Autodesk Fusion 360 part; units mm, degrees
sketch "Sketch3" plane through (0, 0, 0) normal (1, 0, 0) x (0, 1, 0)
  line L0 (0, 0) -> (20, 0)
  line L1 (20, 0) -> (20, 20)
  line L2 (20, 20) -> (0, 20)
  line L3 (0, 20) -> (0, 0)
  dimension "d24" = 20
  dimension "d27" = 20
extrude "Extrude3" add sketch "Sketch3" along normal blind 5
sketch "Sketch4" plane through (5, 0, 0) normal (1, 0, 0) x (0, 1, 0)
  line L0 (0, 20) -> (0, 0)
  line L1 (0, 0) -> (20, 0)
  line L2 (20, 0) -> (20, 20)
  line L3 (20, 20) -> (0, 20)
  line L4 (2, 0) -> (2, 17)
  line L5 (2, 17) -> (10, 17)
  line L6 (10, 17) -> (10, 11)
  line L7 (10, 11) -> (8.5, 11)
  line L8 (8.5, 11) -> (8.5, 5)
  line L9 (8.5, 5) -> (20, 5)
  line L10 (20, 0) -> (2, 0)
  line L11 (20, 0) -> (20, 5)
  dimension "d30" = 8
  dimension "d31" = 2
  dimension "d32" = 6.5
  dimension "d33" = 12
  dimension "d35" = 6
  dimension "d36" = 5
extrude "Extrude4" cut sketch "Sketch4" against normal through all contours L1 L2 L4 L5 L6 L7 L8 L9 L10 L11
fillet "Fillet1" radius 1 7 edges at (2.5, 8.5, 5) (2.5, 10, 17) (2.5, 20, 5) (2.5, 20, 20) (2.5, 0, 20) (2.5, 0, 0) (2.5, 2, 0)
Design review of the part built by this model. Coordinates are the model's own, in mm. A direction names the side the tool comes from. Round coordinates to 2 decimals unless told otherwise and drop trailing zeros. Order: outer loops, then holes, each group sorted by start corner. A loop starts at its lowest first (then second) coordinate and runs counter-clockwise, first axis right, second up.
1) Consider section D-D (z = 4). State the section outline as (x, y) points.
The answers:
outline: (0, 0) - (5, 0) - (5, 2) - (0, 2) - close
2) Consider section C-C (y = 5). State the section outline as (x, z) points.
The answers:
outline: (0, 17) - (5, 17) - (5, 20) - (0, 20) - close
3) Draft analysis for pull direction Z (two halves, no side actions). For faces 6 (the cylindrical face through (2.465, 8.801, 5.285)), 7 (the flat face through (3, 10, 14)), 8 (the flat face through (5, 12, 12)), state which applies: released by +Z, released by -Z, zero draft, split by the parting line, or undercut.
The answers:
face 6: released by -Z
face 7: undercut
face 8: zero draft
4) Machinability: for faces 1 (the cylindrical face through (2.535, 0.301, 19.715)), 2 (the flat face through (0, 12, 12)), 3 (the flat face through (3, 8.5, 9)), 4 (the flat face through (3, 9, 11)), 5 (the flat face through (3, 14, 5)), which of the approach directions +Z, -Z, +X, -X, +Y, -Y give a long, thin tool a straight path to every point of the face, cutting with its end or side? Answer none if there is none.
The answers:
face 1: +Z, +X, -X, -Y
face 2: +Z, -Z, -X, +Y, -Y
face 3: -Z, +X, -X
face 4: +X, -X
face 5: -Z, +X, -X, +Y
5) Consider section A-A (z = 13). State the section outline as (x, y) points.
The answers:
outline: (0, 0) - (5, 0) - (5, 2) - (0, 2) - close; (0, 10) - (5, 10) - (5, 20) - (0, 20) - close
6) For L1, parallel to Y at x = 2.5, z = 14; L2, parallel to Z at x = 0.65, y = 12.5; L3, parallel to Y at x = 1.15, z = 6.5, list the stretches that pass through material, from the lowest coordinate up.
The answers:
L1: y = 0 to 2, 10 to 20
L2: z = 5 to 20
L3: y = 0 to 2, 8.5 to 20
7) Clearance check with flat-ended pins moving along their axes: pin 1 Ø1.5 at (x, y) = (3, 5) entering from -Z; pin 2 Ø1.5 at (x, z) = (2, 4) entering from +Y. State where each tip first meets the part, or that it passes through.
The answers:
pin 1: stops at z = 17
pin 2: stops at y = 2
